from build123d import *

# Parameters (mm, degrees)
SKETCH1_W           = 45
SKETCH1_H           = 42.1
BOSS_EXTRUDE1_DEPTH = 3
SKETCH2_W           = 45
SKETCH2_H           = 3
BOSS_EXTRUDE2_DEPTH = 45
SKETCH4_R           = 11.25
CUT_EXTRUDE1_DEPTH  = 66.871541655
SKETCH5_R           = 1.75
CUT_EXTRUDE2_DEPTH  = 66.871541655
SKETCH6_R           = 1.55
CUT_EXTRUDE3_DEPTH  = 3
BOSS_EXTRUDE3_DEPTH = 2.5


with BuildPart() as part:
    # Sketch1 → Boss-Extrude1 (new body)
    with BuildSketch(Plane(origin=(0, 0, 0), x_dir=(1, 0, 0), z_dir=(0, 1, 0))):
        Rectangle(SKETCH1_W, SKETCH1_H)
    extrude(amount=BOSS_EXTRUDE1_DEPTH)

    # Sketch2 → Boss-Extrude2 (add)
    with BuildSketch(Plane.XZ.offset(-3)):
        with Locations((0, 19.55)):
            Rectangle(SKETCH2_W, SKETCH2_H)
    extrude(amount=-BOSS_EXTRUDE2_DEPTH)

    # Sketch4 → Cut-Extrude1 (cut, through all)
    with BuildSketch(Plane(origin=(0, 0, 18.05), x_dir=(-1, 0, 0), z_dir=(0, 0, -1))):
        with Locations((0, 25.5)):
            Circle(SKETCH4_R)
    extrude(amount=-CUT_EXTRUDE1_DEPTH, mode=Mode.SUBTRACT)

    # Sketch5 → Cut-Extrude2 (cut, through all)
    with BuildSketch(Plane(origin=(0, 0, 18.05), x_dir=(-1, 0, 0), z_dir=(0, 0, -1))):
        with Locations((-15.5, 41)):
            Circle(SKETCH5_R)
        with Locations((15.5, 41)):
            Circle(SKETCH5_R)
        with Locations((15.5, 10)):
            Circle(SKETCH5_R)
        with Locations((-15.5, 10)):
            Circle(SKETCH5_R)
    extrude(amount=-CUT_EXTRUDE2_DEPTH, mode=Mode.SUBTRACT)

    # Sketch6 → Cut-Extrude3 (cut)
    with BuildSketch(Plane(origin=(0, 3, 0), x_dir=(1, 0, 0), z_dir=(0, 1, 0))):
        with Locations(Location((12.5, -10, 0), (0, 0, 270))):
            Circle(SKETCH6_R)
        with Locations(Location((-12.5, -10, 0), (0, 0, 270))):
            Circle(SKETCH6_R)
        with Locations(Location((-12.5, 10, 0), (0, 0, 270))):
            Circle(SKETCH6_R)
        with Locations(Location((12.5, 10, 0), (0, 0, 270))):
            Circle(SKETCH6_R)
    extrude(amount=-CUT_EXTRUDE3_DEPTH, mode=Mode.SUBTRACT)

    # Sketch8 → Boss-Extrude3 (add)
    with BuildSketch(Plane(origin=(22.5, 0, 0), x_dir=(0, 0, -1), z_dir=(1, 0, 0))):
        Polygon((-18.05, 48), (21.05, 3), (-18.05, 3), align=None)
    boss_extrude3 = extrude(amount=-BOSS_EXTRUDE3_DEPTH)

    # Mirror1: Boss-Extrude3 across plane
    add(boss_extrude3.mirror(Plane(origin=(0, 0, 0), x_dir=(0, 0, 1), z_dir=(1, 0, 0))))


solid = part.part
Input: part model. Units: mm. Frame: model coordinates. A direction names the side the tool comes from. Coordinates: 2 decimals unless noted, no trailing zeros. Write each loop counter-clockwise with the first axis right and the second up, starting at its lowest first coordinate (ties: lowest second). Pieces come first, ordered by that corner, then holes. Notation, with made-up numbers: M -1,-23 L 7,-23 A28 cw 7,-1 Z; hole C -18,59.25 d6. An arc over 180 degrees is marked long. Answer as a JSON object with one key per item and string values. Group by question number.
(1) Section C-C on x = 0. Output: boundary loops of the cut face in (y, z).
(2) Section A-A on x = 15.5. Output: boundary loops of the cut face in (y, z), plus the area to 3 significant figures.
(3) Ray query, line 1 along X through (y, z) = (2.2, -10); line 2 along Y through (x, z) = (15.5, 19.2); line 3 along X through (y, z) = (32, 15). Return the intervals inside material, ascending. Write a range as [from, to].
(4) Set-up query: faces 1 (the face through (0, 3, -2)), 2 (the face through (-13.44, 1.52, -11.23)). Return all of +Z, -Z, +X, -X, +Y, -Y with unobstructed straight access to the full face (end or side cutting, diameter ignored); none if empty.
(5) Contact query for flat-ended pins moving along their axis: P1, Ø5.5, axis at x = 15.5, y = 10, coming from the -Z side; P2, Ø19.5, axis at x = -5, z = 5.5, coming from the +Y side; P3, Ø8, axis at x = -17.5, y = 33, coming from the -Z side. Output: stop coordinate, or through.
(6) Section B-B on y = 34.5. Output: boundary loops of the cut face in (x, z).
(7) Mould query, pull axis Z, two halves, no side actions, for faces 3 (the face through (-21.268, 25.815, -1.226)), 4 (the face through (-15.272, 11.735, 19.529)), 5 (the face through (-13.44, 1.52, 8.77)). Classes: pulls with the +Z half, pulls with the -Z half, needs draft (parallel to the pull), parting line crosses it, or undercut.
(8) Section D-D on z = -10.5. Output: boundary loops of the cut face in (x, y), plus the area to 3 significant figures.
Result set:
{
 "1": {"outline": "M 0,-21.05 L 3,-21.05 L 3,18.05 L 14.25,18.05 L 14.25,21.05 L 0,21.05 Z; M 36.75,18.05 L 48,18.05 L 48,21.05 L 36.75,21.05 Z"},
 "2": {"outline": "M 0,-21.05 L 3,-21.05 L 3,18.05 L 8.25,18.05 L 8.25,21.05 L 0,21.05 Z; M 11.75,18.05 L 39.25,18.05 L 39.25,21.05 L 11.75,21.05 Z; M 42.75,18.05 L 48,18.05 L 48,21.05 L 42.75,21.05 Z", "area": "240 mm2"},
 "3": {"line 1": "x = [-22.5, -14.05], [-10.95, 10.95], [14.05, 22.5]", "line 2": "y = [0, 8.25], [11.75, 39.25], [42.75, 48]", "line 3": "x = [-22.5, -20], [20, 22.5]"},
 "4": {"face 1": "-Z, +Y", "face 2": "+Y, -Y"},
 "5": {"P1": "stops at z = 18.05", "P2": "stops at y = 3", "P3": "stops at z = 2.3"},
 "6": {"outline": "M -22.5,6.32 L -20,6.32 L -20,18.05 L -6.75,18.05 L -6.75,21.05 L -22.5,21.05 Z; M 6.75,18.05 L 20,18.05 L 20,6.32 L 22.5,6.32 L 22.5,21.05 L 6.75,21.05 Z"},
 "7": {"face 3": "pulls with the -Z half", "face 4": "needs draft", "face 5": "undercut"},
 "8": {"outline": "M -22.5,0 L -13.97,0 L -13.97,3 L -20,3 L -20,15.14 L -22.5,15.14 Z; M -11.03,0 L 11.03,0 L 11.03,3 L -11.03,3 Z; M 13.97,0 L 22.5,0 L 22.5,15.14 L 20,15.14 L 20,3 L 13.97,3 Z", "area": "178 mm2"}
}
